Could you check a few things on this model? Use its own coordinates, in mm. Coordinates: 2 decimals unless noted, no trailing zeros. Loops run counter-clockwise (first coordinate to the right, second up) from the corner with the lowest first, then second, coordinate; pieces in that order, holes last. Notation, with made-up numbers: M 35.25,67.5 L 83.25,67.5 A25 ccw 83.25,84.5 Z; hole C 79,79 d3. An arc over 180 degrees is marked long. Write each question's results on one line, items separated by ' | '.
Autodesk Inventor part; units mm, degrees
ref_plane "YZ Plane" through (0, 0, 0) normal (1, 0, 0) x (0, 1, 0)
ref_plane "XZ Plane" through (0, 0, 0) normal (0, 1, 0) x (-1, 0, 0)
ref_plane "XY Plane" through (0, 0, 0) normal (0, 0, 1) x (1, 0, 0)
sketch "Sketch1" plane through (0, 0, 0) normal (0, 1, 0) x (-1, 0, 0)
  line L0 (0, 0) -> (205, 0)
  line L1 (205, 0) -> (205, 290)
  line L2 (205, 290) -> (0, 290)
  line L3 (0, 290) -> (0, 0)
  line L4 (0, 290) -> (50, 290)
  line L5 (50, 290) -> (50, 297.4)
  line L6 (50, 297.4) -> (0, 297.4)
  line L7 (0, 297.4) -> (0, 290)
  line L8 (205, 0) -> (197.5, 0)
  line L9 (197.5, 0) -> (197.5, 17.325)
  circle A0 centre (197.5, 17.325) radius 1.675
  line L10 (197.5, 17.325) -> (197.5, 154.225)
  line L11 (197.5, 154.225) -> (197.5, 167.775)
  circle A1 centre (197.5, 167.775) radius 1.675
  line L12 (197.5, 167.775) -> (197.5, 283.785)
  circle A2 centre (197.5, 283.785) radius 1.675
  line L13 (197.5, 167.775) -> (197.5, 146.525)
  line L14 (197.5, 146.525) -> (118.5, 146.525)
  circle A3 centre (118.5, 146.525) radius 1.675
  line L15 (197.5, 283.785) -> (72.5, 283.785)
  circle A4 centre (72.5, 283.785) radius 1.675
  line L16 (197.5, 17.325) -> (197.5, 38.875)
  line L17 (197.5, 38.875) -> (32.5, 38.875)
  line L18 (32.5, 38.875) -> (32.5, 35.525)
  circle A5 centre (32.5, 35.525) radius 1.675
  dimension "d0" = 205
  dimension "d1" = 290
  dimension "d2" = 50
  dimension "d3" = 7.4
  dimension "d4" = 7.5
  dimension "d5" = 17.325
  dimension "d6" = 3.35
  dimension "d7" = 136.9
  dimension "d8" = 13.55
  dimension "d9" = 3.35
  dimension "d10" = 116.01
  dimension "d11" = 3.35
  dimension "d12" = 21.25
  dimension "d13" = 79
  dimension "d14" = 3.35
  dimension "d15" = 125
  dimension "d16" = 3.35
  dimension "d17" = 21.55
  dimension "d18" = 165
  dimension "d24" = 3.35
extrude "Extrusion2" add sketch "Sketch1" along normal blind 2
properties part number "base_main_pcb"
(1) Please list where these lines run through material, in increasing order: probe 1 along Z at (x, y) = (-197.5, 1.1); probe 2 along Z at (x, y) = (-72.5, 0.5); probe 3 along Z at (x, y) = (-32.5, 0.9). Write a range as from..to.
Reported:
probe 1: z = 0..15.65, 19..166.1, 169.45..282.11, 285.46..290 | probe 2: z = 0..282.11, 285.46..290 | probe 3: z = 0..33.85, 37.2..297.4
(2) Imagine slicing it at B-B, the plane x = -77.5. List the corners of the cut face in (y, z) for me.
Reported:
outline: M 0,0 L 2,0 L 2,290 L 0,290 Z
(3) Imagine slicing it at A-A, the plane y = 1.3. List the corners of the cut face in (x, z) for me (3 decimals).
Reported:
outline: M -205,0 L 0,0 L 0,297.4 L -50,297.4 L -50,290 L -205,290 Z; hole C -197.5,17.325 d3.35; hole C -197.5,167.775 d3.35; hole C -197.5,283.785 d3.35; hole C -118.5,146.525 d3.35; hole C -72.5,283.785 d3.35; hole C -32.5,35.525 d3.35
(4) If we mould it in two halves opening along Y, with no side actions, what happens to faces 1 (the flat face through (-101, 0, 151)), 2 (the flat face through (-101, 2, 151))? For each: released by +Y, released by -Y, zero draft, split by the parting line, or undercut.
Reported:
face 1: released by -Y | face 2: released by +Y
